Check sheet for the modelled part. Datum: model origin and axes. Units: mm. A direction names the side the tool comes from. Give positions to 0.01 mm unless a question says otherwise; leave off trailing zeros. Order: outer loops, then holes, each group sorted by start corner. A loop starts at its lowest first (then second) coordinate and runs counter-clockwise, first axis right, second up.
Item 1: Access from +Z, -Z, +X, -X, +Y, -Y to the whole of each face (thin tool, end or side, straight path). Record for faces 5 (the flat face through (12.7, 2.5, 5)), 6 (the flat face through (13.08, 2.5, 4.5)), 7 (the flat face through (11, 5.5, 0)), 8 (the cylindrical face through (-12, 2, 0)), 9 (the cylindrical face through (13.819, 0.517, 3.732)).
Item 2: Gauge pin test, flat ends, axial feed: P1, Ø1.5, axis at x = 12.5, z = -5, coming from the +Y side; P2, Ø0.6, axis at x = 14, y = 1.5, coming from the +Z side; P3, Ø1.5, axis at x = 8.5, y = 3.5, coming from the +Z side; P4, Ø4, axis at y = 4.5, z = -7.5, coming from the -X side. Record the tip position at first contact, or that the pin passes through.
Item 3: Sectioned sample at A-A on x = 0. Record the boundary of the cut face in (y, z).
Item 4: Material ranges on line 1 along Z through (x, y) = (0, 2.5); line 2 along Z through (x, y) = (9.75, 4.25); line 3 along X through (y, z) = (4.25, -8.25), recorded low to high.
Item 5: Sectioned sample at D-D on y = -0.5. Record the boundary of the cut face in (x, z).
Item 6: Release check for a two-part mould opening along Z. For faces 1 (the cylindrical face through (-2.38, 2.46, -10.74)), 2 (the flat face through (11, -0.5, 0)), 3 (the flat face through (14, 3, 4)), 4 (the flat face through (14, 3, -2.5)) record: released by +Z, released by -Z, zero draft, split by the parting line, or undercut.
Item 7: Sectioned sample at B-B on y = 2.5. Record the boundary of the cut face in (x, z).
Item 8: Sectioned sample at C-C on z = -4.25. Record the boundary of the cut face in (x, y), and give its area (3 significant figures).
Solid Edge part; units mm, degrees
sketch "Sketch1" plane through (0, 0, 0) normal (0, -1, 0) x (1, 0, 0)
  circle A0 centre (0, 0) radius 12
  circle A1 centre (0, 0) radius 11
extrude "Protrusion1" add sketch "Sketch1" against normal blind 5
sketch "Sketch2" plane through (0, 0, 0) normal (0, 0, 1) x (1, 0, 0)
  line L0 (11, 6) -> (11, -1)
  line L1 (11, -1) -> (13, -1)
  line L2 (13, -1) -> (13, 0.2087)
  line L3 (13, 6) -> (13, 4.7913)
  line L4 (11, 6) -> (13, 6)
  arc A0 (13, 0.2087) -> (13, 4.7913) centre (14, 2.5) ccw
  dimension "D1" = 11
  dimension "D2" = 14
extrude "Protrusion2" add sketch "Sketch2" along normal mid plane 5
sketch "Sketch3" plane through (13.75, 2.5, 2.5) normal (0, 0, 1) x (1, 0, 0)
  circle A0 centre (0.3296, 0) radius 2
extrude "Protrusion3" add sketch "Sketch3" along normal mid plane 5
sketch "Sketch4" plane through (14.0796, 2.5, 5) normal (0, 0, 1) x (1, 0, 0)
  line L0 (-1, 2.5) -> (1, 2.5)
  line L1 (1, 2.5) -> (1, -2.5)
  line L2 (1, -2.5) -> (-1, -2.5)
  line L3 (-1, -2.5) -> (-1, 2.5)
  dimension "D1" = 1
  dimension "D2" = 1
extrude "ExtrudedCutout_1" cut sketch "Sketch4" against normal blind 1
properties material "Aluminum, 1350"
Report:
1. face 5: +Z, +X, +Y, -Y
1. face 6: +Z, +Y, -Y
1. face 7: +Z, -Z, -X, +Y
1. face 8: +Y, -Y
1. face 9: +Z
2. P1: passes through
2. P2: stops at z = 4
2. P3: stops at z = 9.16
2. P4: stops at x = -10.67
3. outline: (0, -12) - (5, -12) - (5, -11) - (0, -11) - close; (0, 11) - (5, 11) - (5, 12) - (0, 12) - close
4. line 1: z = -12 to -11, 11 to 12
4. line 2: z = -7 to -5.09, 5.09 to 7
4. line 3: x = -8.71 to -7.28, 7.28 to 8.71
5. outline: (11, -2.5) - (13, -2.5) - (13, 2.5) - (11, 2.5) - close
6. face 1: undercut
6. face 2: zero draft
6. face 3: released by +Z
6. face 4: released by -Z
7. outline: (11.74, -2.5) - (16.5, -2.5) - (16.5, 2.5) - (16.08, 2.5) - (16.08, 5) - (15.08, 5) - (15.08, 4) - (13.08, 4) - (13.08, 5) - (12.08, 5) - (12.08, 2.5) - (11.74, 2.5) arc R12 ccw (long way) to start; hole circle Ø22 at (0, 0)
8. outline: (-11.22, 0) - (-10.15, 0) - (-10.15, 5) - (-11.22, 5) - close; (10.15, 0) - (11.22, 0) - (11.22, 5) - (10.15, 5) - close
8. area: 10.8 mm2
